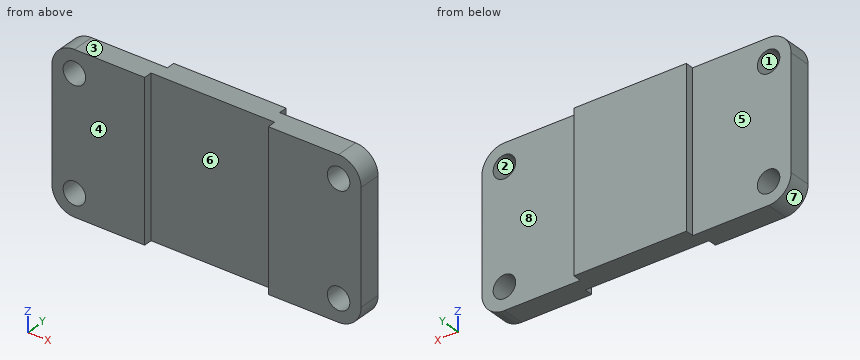
from build123d import *

# Parameters (mm, degrees)
IZIM1_R                     = 40
Y_KSEKLIK_EKSTR_ZYON1_DEPTH = 80
IZIM2_W                     = 440
IZIM2_H                     = 30
KES_EKSTR_ZYON1_DEPTH       = 789.986691903
IZIM3_W                     = 400
IZIM3_H                     = 30
Y_KSEKLIK_EKSTR_ZYON2_DEPTH = 560


with BuildPart() as part:
    # Çizim1 → Yükseklik-Ekstrüzyon1 (new body)
    with BuildSketch(Plane(origin=(0, 0, 0), x_dir=(1, 0, 0), z_dir=(0, 1, 0))):
        with BuildLine():
            Line((-470, -280), (470, -280))
            ThreePointArc((470, -280), (526.568542495, -256.568542495), (550, -200))
            Line((550, -200), (550, 200))
            ThreePointArc((550, 200), (526.568542495, 256.568542495), (470, 280))
            Line((470, 280), (-470, 280))
            ThreePointArc((-470, 280), (-526.568542495, 256.568542495), (-550, 200))
            Line((-550, 200), (-550, -200))
            ThreePointArc((-550, -200), (-526.568542495, -256.568542495), (-470, -280))
        make_face()
        with Locations(Location((-470, 200, 0), (0, 0, 270))):
            Circle(IZIM1_R, mode=Mode.SUBTRACT)
        with Locations(Location((-470, -200, 0), (0, 0, 270))):
            Circle(IZIM1_R, mode=Mode.SUBTRACT)
        with Locations(Location((470, -200, 0), (0, 0, 270))):
            Circle(IZIM1_R, mode=Mode.SUBTRACT)
        with Locations(Location((470, 200, 0), (0, 0, 270))):
            Circle(IZIM1_R, mode=Mode.SUBTRACT)
    extrude(amount=Y_KSEKLIK_EKSTR_ZYON1_DEPTH)

    # Çizim2 → Kes-Ekstrüzyon1 (cut, through all)
    with BuildSketch(Plane.XY.offset(280)):
        with Locations((0, 15)):
            Rectangle(IZIM2_W, IZIM2_H)
    extrude(amount=-KES_EKSTR_ZYON1_DEPTH, mode=Mode.SUBTRACT)

    # Çizim3 → Yükseklik-Ekstrüzyon2 (add)
    with BuildSketch(Plane.XY.offset(280)):
        with Locations((0, 95)):
            Rectangle(IZIM3_W, IZIM3_H)
    extrude(amount=-Y_KSEKLIK_EKSTR_ZYON2_DEPTH)


solid = part.part
The model under review builds one solid part; all positions refer to its coordinate system, in mm. Face numbers are marked on the shaded views. A direction names the side the tool comes from. Give positions to 0.01 mm unless a question says otherwise; leave off trailing zeros. Order: outer loops, then holes, each group sorted by start corner. A loop starts at its lowest first (then second) coordinate and runs counter-clockwise, first axis right, second up. Notation, with made-up numbers: M 33,23 L 79,23 A20 cw 79,56 Z; hole C 8.25,5.25 d4. An arc over 180 degrees is marked long. One line per question, with ' | ' between items. Start each with the question number.
1) For the marked faces 5, 6, 7 and 8, list the 3-axis set-ups (+Z, -Z, +X, -X, +Y, -Y) from which the entire face can be reached by the end or side of a thin tool; tool diameter is ignored.
2) Consider section A-A, the plane y = 14.5. Give the boundary of the cut face in (x, z).
3) Consider section B-B, the plane y = 63.5. Give the boundary of the cut face in (x, z).
4) Mouldability with a two-part tool opening along Z and no side actions: class the marked faces 1, 2, 3 and 4 as pulls with the +Z half, pulls with the -Z half, needs draft (parallel to the pull), parting line crosses it, or undercut.
5) Consider section D-D, the plane x = -49.5. Give the boundary of the cut face in (y, z), then the cut area to 3 significant figures.
6) Consider section C-C, the plane z = 114. Give the boundary of the cut face in (x, y).
7) Clearance check with flat-ended pins moving along their axes: P1, Ø10, axis at x = -277, z = -138.5, coming from the -Y side; P2, Ø8, axis at x = -134.5, z = -149.5, coming from the -Y side; P3, Ø24, axis at y = 99, z = -69.5, coming from the -X side. State where each tip first meets the part, or that it passes through.
8) Wall thickness on L1, parallel to X at y = 42, z = 200; L2, parallel to X at y = 24, z = 200; L3, parallel to X at y = 20.5, z = 78: over which ranges is each line inside the solid? List them lowest first. Write a range as from..to.
Found:
1) face 5: +Z, -Z, -X, +Y | face 6: +Z, -Z, -Y | face 7: -Z, -X, +Y, -Y | face 8: +Z, -Z, +X, +Y
2) outline: M -550,-200 A80 ccw -470,-280 L -220,-280 L -220,280 L -470,280 A80 ccw -550,200 Z; M 220,-280 L 470,-280 A80 ccw 550,-200 L 550,200 A80 ccw 470,280 L 220,280 Z; hole C -470,-200 d80; hole C -470,200 d80; hole C 470,-200 d80; hole C 470,200 d80
3) outline: M -550,-200 A80 ccw -470,-280 L 470,-280 A80 ccw 550,-200 L 550,200 A80 ccw 470,280 L -470,280 A80 ccw -550,200 Z; hole C -470,-200 d80; hole C -470,200 d80; hole C 470,-200 d80; hole C 470,200 d80
4) face 1: undercut | face 2: undercut | face 3: pulls with the +Z half | face 4: needs draft
5) outline: M 30,-280 L 110,-280 L 110,280 L 30,280 Z | area: 44,800 mm²
6) outline: M -550,0 L -220,0 L -220,30 L 220,30 L 220,0 L 550,0 L 550,80 L 200,80 L 200,110 L -200,110 L -200,80 L -550,80 Z
7) P1: stops at y = 0 | P2: stops at y = 30 | P3: stops at x = -200
8) L1: x = -550..-510, -430..430, 510..550 | L2: x = -550..-510, -430..-220, 220..430, 510..550 | L3: x = -550..-220, 220..550
